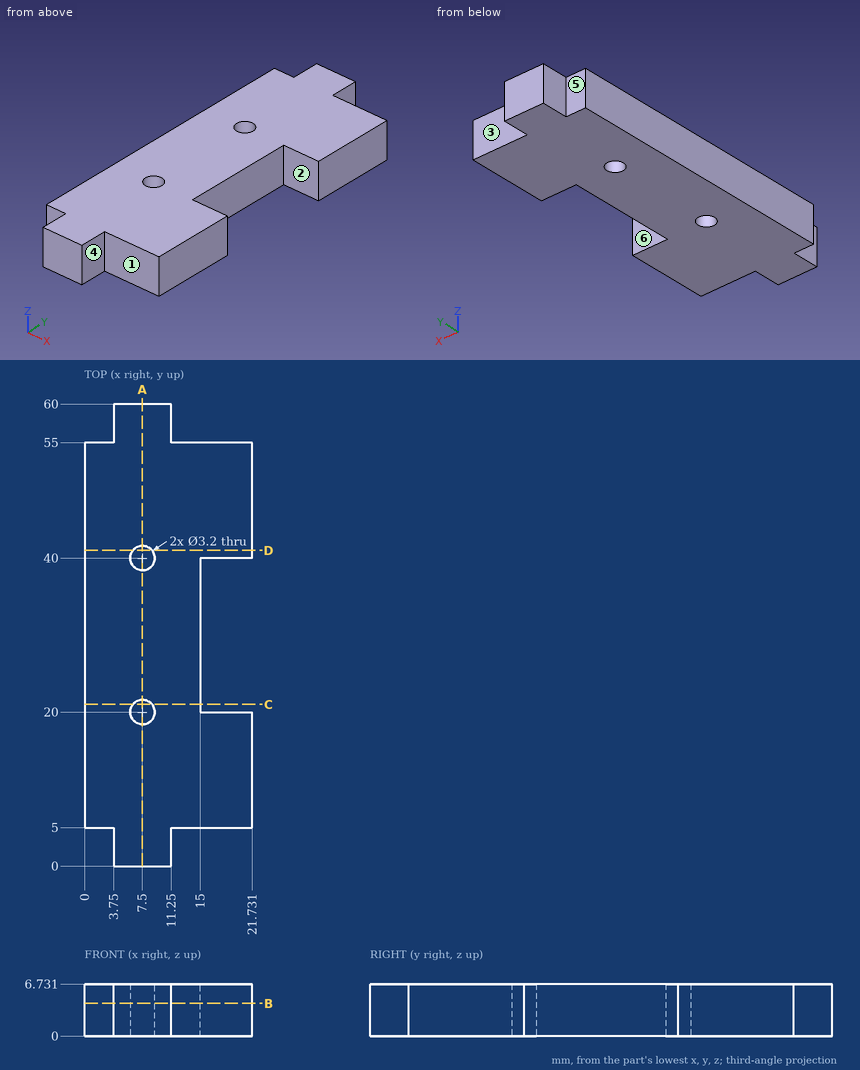
Part print with two shaded views. Sizes in mm from the minimum x, y, z corner. A direction names the side the tool comes from. Coordinates: 2 decimals unless noted, no trailing zeros. Loops run counter-clockwise (first coordinate to the right, second up) from the corner with the lowest first, then second, coordinate; pieces in that order, holes last. Notation, with made-up numbers: (-8, 69.5) - (15, 69.5) arc R14 ccw to (15, 91.5) - close; hole circle Ø11 at (-9, 89). An arc over 180 degrees is marked (long way). Write each question's results on one line, items separated by ' | '. Start each with the question number.
Q1. Drop flat-ended pins along their axis: pin 1 Ø3 at (x, z) = (2.5, 4.5) entering from +Y; pin 2 Ø1.9 at (x, z) = (1.5, 2) entering from -Y; pin 3 Ø2.5 at (y, z) = (3.5, 2) entering from +X; pin 4 Ø1.5 at (y, z) = (57, 2) entering from -X. Give the stop position or say it passes through.
Q2. Two-plate mould, pull along Y, no slides. Class the marked faces 1, 2 and 3: +Y half, -Y half, draft (parallel to the pull), parting line (faces both ways), or undercut.
Q3. Probe line 1 along Y through (x, z) = (7.5, 2.5); line 2 along Y through (x, z) = (20.5, 3.5); line 3 along Y through (x, z) = (14.75, 3). List the from-to ranges inside material, lowest first.
Q4. Slice it at A-A on x = 7.5. Give the cut face in (y, z), and give its area (3 significant figures).
Q5. Slice it at D-D on y = 41. Give the cut face in (x, z), and give its area (3 significant figures).
Q6. Slice it at B-B on z = 4.25. Give the cut face in (x, y), and give its area (3 significant figures).
Q7. Slice it at C-C on y = 21. Give the cut face in (x, z), and give its area (3 significant figures).
Q8. Which spindle directions (+Z, -Z, +X, -X, +Y, -Y) get a long thin tool onto all of the face, cutting with end or side? Do the marked faces 4, 5 and 6. Say none if no direction does.
Answer:
1) pin 1: stops at y = 60 | pin 2: stops at y = 5 | pin 3: stops at x = 11.25 | pin 4: stops at x = 3.75
2) face 1: -Y half | face 2: undercut | face 3: +Y half
3) line 1: y = 0 to 18.4, 21.6 to 38.4, 41.6 to 60 | line 2: y = 5 to 20, 40 to 55 | line 3: y = 5 to 55
4) outline: (0, 0) - (18.4, 0) - (18.4, 6.73) - (0, 6.73) - close; (21.6, 0) - (38.4, 0) - (38.4, 6.73) - (21.6, 6.73) - close; (41.6, 0) - (60, 0) - (60, 6.73) - (41.6, 6.73) - close | area: 361 mm2
5) outline: (0, 0) - (6.25, 0) - (6.25, 6.73) - (0, 6.73) - close; (8.75, 0) - (21.73, 0) - (21.73, 6.73) - (8.75, 6.73) - close | area: 129 mm2
6) outline: (0, 5) - (3.75, 5) - (3.75, 0) - (11.25, 0) - (11.25, 5) - (21.73, 5) - (21.73, 20) - (15, 20) - (15, 40) - (21.73, 40) - (21.73, 55) - (11.25, 55) - (11.25, 60) - (3.75, 60) - (3.75, 55) - (0, 55) - close; hole circle Ø3.2 at (7.5, 20); hole circle Ø3.2 at (7.5, 40) | area: 1,010 mm2
7) outline: (0, 0) - (6.25, 0) - (6.25, 6.73) - (0, 6.73) - close; (8.75, 0) - (15, 0) - (15, 6.73) - (8.75, 6.73) - close | area: 84.2 mm2
8) face 4: +Z, -Z, +X, -Y | face 5: +Z, -Z, -X, +Y | face 6: +Z, -Z, +X
